Work out the finished part from the listing and answer in its coordinate system (mm). A direction names the side the tool comes from. Coordinates: 2 decimals unless noted, no trailing zeros. Order: outer loops, then holes, each group sorted by start corner. A loop starts at its lowest first (then second) coordinate and runs counter-clockwise, first axis right, second up. Notation, with made-up numbers: (24.25, 5.5) -> (43.25, 5.5) arc R20 cw to (43.25, 43.5) -> close; hole circle Ø11 at (76.5, 76.25). An arc over 180 degrees is marked (long way). Use one line per item in the form item = value.
from build123d import *

# Parameters (mm, degrees)
BOSS_EXTRUDE1_DEPTH = 1.524
CUT_EXTRUDE1_DEPTH  = 1.524
CUT_EXTRUDE2_DEPTH  = 1.524


with BuildPart() as part:
    # Sketch1 → Boss-Extrude1 (new body)
    with BuildSketch(Plane.XY):
        with BuildLine():
            Line((-18.109082737, 18.651136583), (-40.403888228, -0.992394741))
            ThreePointArc((-40.403888228, -0.992394741), (-42.395698567, -4.050724761), (-41.491876636, -7.586795582))
            ThreePointArc((-41.491876636, -7.586795582), (-40.996783491, -7.860427406), (-40.456184155, -7.693862236))
            Line((-40.456184155, -7.693862236), (-27.338891186, 3.372084587))
            Line((-27.338891186, 3.372084587), (-26.367560741, 2.220467499))
            Line((-26.367560741, 2.220467499), (-39.509764326, -8.866336125))
            ThreePointArc((-39.509764326, -8.866336125), (-39.764677025, -9.366363056), (-39.585096423, -9.898113208))
            Line((-39.585096423, -9.898113208), (-36.909039408, -12.923145527))
            ThreePointArc((-36.909039408, -12.923145527), (-36.096292723, -14.255273478), (-36.065454443, -15.815456497))
            ThreePointArc((-36.065454443, -15.815456497), (-38.919913552, -19.419117177), (-40.970693325, -23.533556316))
            ThreePointArc((-40.970693325, -23.533556316), (-85.68561882, -29.806279301), (-109.164446531, -68.374611713))
            ThreePointArc((-109.164446531, -68.374611713), (-86.824997617, -79.693885154), (-62.075353147, -75.868701805))
            ThreePointArc((-62.075353147, -75.868701805), (-53.793448225, -74.248732285), (-46.732322194, -69.627612338))
            ThreePointArc((-46.732322194, -69.627612338), (-43.045880581, -69.354101873), (-39.440165524, -68.539559875))
            ThreePointArc((-39.440165524, -68.539559875), (-30.674096062, -56.183483706), (-28.287271549, -41.22288008))
            ThreePointArc((-28.287271549, -41.22288008), (-18.354497785, -42.11718557), (-8.478792941, -40.727858108))
            Line((-8.478792941, -40.727858108), (-28.809143223, -16.540912603))
            Line((-28.809143223, -16.540912603), (-27.655597936, -15.571510358))
            Line((-27.655597936, -15.571510358), (-6.888329643, -40.281661868))
            ThreePointArc((-6.888329643, -40.281661868), (-2.393348388, -38.654039316), (1.896097193, -36.543430812))
            ThreePointArc((1.896097193, -36.543430812), (14.669066503, -20.423756748), (13.224183609, 0.092211431))
            ThreePointArc((13.224183609, 0.092211431), (12.94908113, 2.915517355), (15.164401866, 4.687265575))
            ThreePointArc((15.164401866, 4.687265575), (15.618518122, 4.953772723), (15.791401816, 5.451124573))
            Line((15.791401816, 5.451124573), (15.559206878, 18.186922579))
            Line((15.559206878, 18.186922579), (17.065612654, 18.214399421))
            Line((17.065612654, 18.214399421), (17.255673973, 7.790267081))
            ThreePointArc((17.255673973, 7.790267081), (17.649146232, 7.159803879), (18.390670497, 7.209261245))
            ThreePointArc((18.390670497, 7.209261245), (24.284101701, 9.245801019), (30.497638202, 8.724274642))
            ThreePointArc((30.497638202, 8.724274642), (31.008729101, 8.935857556), (31.220713438, 9.446782089))
            Line((31.220713438, 9.446782089), (31.227755152, 18.421680855))
            Line((31.227755152, 18.421680855), (32.734160928, 18.420716756))
            Line((32.734160928, 18.420716756), (32.727120315, 9.492749656))
            ThreePointArc((32.727120315, 9.492749656), (32.938701818, 8.981090412), (33.450193713, 8.769104665))
            Line((33.450193713, 8.769104665), (36.00103405, 8.76910061))
            Line((36.00103405, 8.76910061), (39.593571682, 7.750734608))
            ThreePointArc((39.593571682, 7.750734608), (37.634153074, 11.103388424), (36.980980252, 14.931308767))
            ThreePointArc((36.980980252, 14.931308767), (37.32973025, 16.244488278), (38.290753444, 17.204957649))
            ThreePointArc((38.290753444, 17.204957649), (40.689125585, 17.029816962), (42.926139447, 16.147415598))
            ThreePointArc((42.926139447, 16.147415598), (42.166781774, 18.73974704), (42.447864883, 21.426343152))
            ThreePointArc((42.447864883, 21.426343152), (39.616652478, 30.812755933), (31.670318465, 36.555254025))
            ThreePointArc((31.670318465, 36.555254025), (30.869545829, 36.286258041), (30.870312564, 35.441512478))
            Line((30.870312564, 35.441512478), (35.931597573, 28.422287011))
            Line((35.931597573, 28.422287011), (34.710083257, 27.541099888))
            Line((34.710083257, 27.541099888), (28.048154351, 36.779585234))
            ThreePointArc((28.048154351, 36.779585234), (26.749368414, 37.368488779), (25.351600254, 37.085829151))
            ThreePointArc((25.351600254, 37.085829151), (20.481432232, 44.59849919), (16.594043627, 52.663668593))
            ThreePointArc((16.594043627, 52.663668593), (19.678771518, 42.480420055), (25.014453648, 33.274737399))
            ThreePointArc((25.014453648, 33.274737399), (24.630642645, 31.475856238), (25.014447927, 29.676973856))
            ThreePointArc((25.014447927, 29.676973856), (24.481307432, 30.159012342), (23.8292382, 30.461345943))
            ThreePointArc((23.8292382, 30.461345943), (20.663534908, 33.163038536), (17.321589669, 35.643405891))
            ThreePointArc((17.321589669, 35.643405891), (15.461285039, 36.273044307), (13.767992132, 35.278088539))
            ThreePointArc((13.767992132, 35.278088539), (10.258583377, 26.939942946), (8.042121541, 18.169086735))
            ThreePointArc((8.042121541, 18.169086735), (4.666584105, 15.017884217), (1.052433145, 12.143472427))
            ThreePointArc((1.052433145, 12.143472427), (-2.67031295, 12.596290492), (-6.419385375, 12.504974353))
            ThreePointArc((-6.419385375, 12.504974353), (-8.511533948, 12.739347863), (-9.521951073, 14.586257126))
            ThreePointArc((-9.521951073, 14.586257126), (-12.55527012, 19.280991071), (-18.109082737, 18.651136583))
        make_face()
    extrude(amount=BOSS_EXTRUDE1_DEPTH)

    # Sketch2 → Cut-Extrude1 (cut)
    with BuildSketch(Plane(origin=(0, 0, 0), x_dir=(-1, 0, 0), z_dir=(0, 0, -1))):
        Polygon((-7.412304672, -34.333896752), (12.756455248, -10.335886692), (11.589770834, -9.355364649), (-8.578989086, -33.353374708), align=None)
    extrude(amount=-CUT_EXTRUDE1_DEPTH, mode=Mode.SUBTRACT)

    # Sketch3 → Cut-Extrude2 (cut)
    with BuildSketch(Plane(origin=(0, 0, 0), x_dir=(-1, 0, 0), z_dir=(0, 0, -1))):
        Polygon((92.239440666, -85.195390194), (57.69869779, -66.269905982), (56.966391259, -67.606432504), (91.507134135, -86.531916716), align=None)
        Polygon((113.568916303, -69.443616856), (65.468307652, -51.334573831), (64.931342073, -52.760843078), (113.031950724, -70.869886103), align=None)
        Polygon((103.892541474, -43.556614737), (61.98194232, -33.329554282), (61.620655619, -34.810110907), (103.531254772, -45.037171362), align=None)
    extrude(amount=-CUT_EXTRUDE2_DEPTH, mode=Mode.SUBTRACT)


solid = part.part
(1) Section D-D on x = -51.5 is taken. Write down the section's boundary in (y, z), plus the area to 3 significant figures.
Data:
outline = (-73.16, 0) -> (-21.39, 0) -> (-21.39, 1.52) -> (-73.16, 1.52) -> close
area = 78.9 mm²
(2) Section A-A on x = -88.5 is taken. Write down the section's boundary in (y, z).
Data:
outline = (-79.39, 0) -> (-61.63, 0) -> (-61.63, 1.52) -> (-79.39, 1.52) -> close; (-60.01, 0) -> (-41.37, 0) -> (-41.37, 1.52) -> (-60.01, 1.52) -> close; (-39.8, 0) -> (-31.79, 0) -> (-31.79, 1.52) -> (-39.8, 1.52) -> close
(3) This flat-tipped pin is pushed along its axis until it touches: P1, Ø0.8, axis at x = 35, z = 0.5, coming from the -Y side. Where does it stop, or does it pass through?
Data:
P1 = 8.77
(4) Straight lines are drawn through the part: line 1 along Y through (x, z) = (-94, 0.35); line 2 along X through (y, z) = (-20, 0.9); line 3 along Y through (x, z) = (-85, 1.25). For each, find the intervals that lie inside material, in ascending order.
Data:
line_1 = -77.87 to -63.7, -62.08 to -42.71, -41.14 to -36.58
line_2 = -39.28 to -25.9, -23.93 to -4.63, -2.64 to 14.8
line_3 = -79.94 to -60.32, -58.69 to -40.52, -38.95 to -29.36
(5) The mould has two halves that part along Y. Classify faces 1 (the cylindrical face through (-53.9, -74.29, 0.75)), 2 (the flat face through (-80.72, -39.47, 0.75)), 3 (the flat face through (-39, -28, 1.524)): released by +Y, released by -Y, zero draft, split by the parting line, or undercut.
Data:
face_1 = released by -Y
face_2 = undercut
face_3 = zero draft
(6) Which of the six approach directions +Z, -Z, +X, -X, +Y, -Y give full straight-line access (tool end or side, diameter ignored) to faces 4 (the flat face through (-2.14, -20.6, 0.75)), 5 (the cylindrical face through (-2.5, -38.7, 0.8)), 6 (the cylindrical face through (4.716, 15.06, 0.751))?
Data:
face_4 = +Z, -Z
face_5 = +Z, -Z, +X, -Y
face_6 = +Z, -Z, +Y
(7) Section C-C on x = 10 is taken. Write down the section's boundary in (y, z), plus the area to 3 significant figures.
Data:
outline = (-29.41, 0) -> (26.15, 0) -> (26.15, 1.52) -> (-29.41, 1.52) -> close
area = 84.7 mm²
(8) Section B-B on y = -56.5 is taken. Write down the section's boundary in (x, z), plus the area to 3 significant figures.
Data:
outline = (-106.51, 0) -> (-79.19, 0) -> (-79.19, 1.52) -> (-106.51, 1.52) -> close; (-74.86, 0) -> (-30.81, 0) -> (-30.81, 1.52) -> (-74.86, 1.52) -> close
area = 109 mm²
